Work out the finished part from the listing and answer in its coordinate system (mm). Give positions to 0.01 mm unless a question says otherwise; leave off trailing zeros. Loops run counter-clockwise (first coordinate to the right, second up) from the corner with the lowest first, then second, coordinate; pieces in that order, holes last. Notation, with made-up numbers: M -17,1 L -2,1 A14 ccw -2,18 Z; hole C 80,-15.75 d2. An arc over 180 degrees is marked long. Answer as a JSON object with one key per item and string values. Group by question number.
Autodesk Inventor part; units mm, degrees
ref_plane "YZ Plane" through (0, 0, 0) normal (1, 0, 0) x (0, 1, 0)
ref_plane "XZ Plane" through (0, 0, 0) normal (0, 1, 0) x (-1, 0, 0)
ref_plane "XY Plane" through (0, 0, 0) normal (0, 0, 1) x (1, 0, 0)
sketch "Sketch1" plane through (0, 0, 0) normal (0, 1, 0) x (-1, 0, 0)
  line L0 (-50, 50) -> (50, 50)
  line L1 (50, 50) -> (50, -50)
  line L2 (50, -50) -> (-50, -50)
  line L3 (-50, -50) -> (-50, 50)
  line L4 (-50, 50) -> (50, -50) construction
  line L5 (50, 50) -> (-50, -50) construction
  point P0 (0, 0)
  dimension "d0" = 100
  dimension "d1" = 100
extrude "Extrusion1" add sketch "Sketch1" along normal blind 3
sketch "Sketch2" plane through (0, 3, 0) normal (0, 1, 0) x (1, 0, 0)
  point P0 (0, 0)
  point P1 (0, 0)
hole "Hole1" at (0, 3, 0) direction (0, -1, 0) diameter 76.3 end through all
sketch "Sketch3" plane through (0, 3, 0) normal (0, 1, 0) x (1, 0, 0)
  line L0 (-50, -50) -> (50, -50)
  line L1 (-50, 50) -> (-50, -50)
  point P0 (0, 0)
  point P1 (-37.5, -37.5)
  point P2 (37.5, -37.5)
  point P3 (0, 0)
  point P4 (37.5, 37.5)
  point P5 (0, 0)
  point P6 (-37.5, 37.5)
  point P7 (0, 0)
  dimension "d18" = 12.5
  dimension "d19" = 12.5
  dimension "d22" = 360
hole "Hole2" at (-37.5, 3, 37.5) at (-37.5, 3, -37.5) at (37.5, 3, -37.5) at (37.5, 3, 37.5) direction (0, -1, 0) diameter 5 end through all
properties part number "Plant Panel" material "Aluminum 6061"
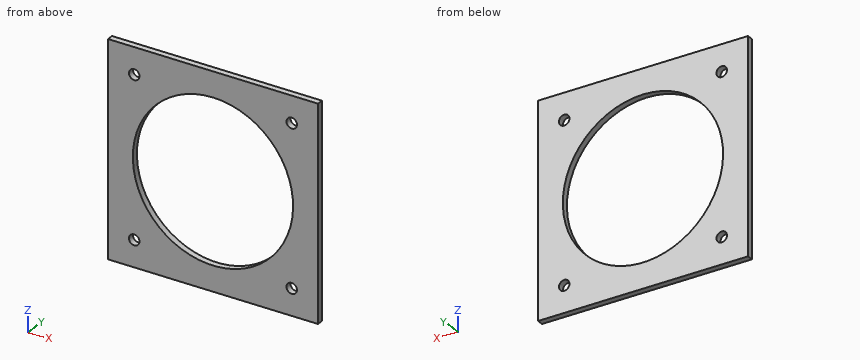
Item 1: A cutting plane is placed at B-B (x = 0). Determine the outline of the cut face in (y, z).
Item 2: A cutting plane is placed at A-A (z = 32.5). Determine the outline of the cut face in (x, y).
Item 3: Find the intervals of material crossed by probe 1 along X at (y, z) = (0.8, 39.5); probe 2 along X at (y, z) = (2.6, 0); probe 3 along X at (y, z) = (2, 13.5), in increasing order. Write a range as [from, to].
Item 4: A cutting plane is placed at C-C (y = 0.75). Determine the outline of the cut face in (x, z).
The answers:
{
 "1": {"outline": "M 0,-50 L 3,-50 L 3,-38.15 L 0,-38.15 Z; M 0,38.15 L 3,38.15 L 3,50 L 0,50 Z"},
 "2": {"outline": "M -50,0 L -19.98,0 L -19.98,3 L -50,3 Z; M 19.98,0 L 50,0 L 50,3 L 19.98,3 Z"},
 "3": {"probe 1": "x = [-50, -39], [-36, 36], [39, 50]", "probe 2": "x = [-50, -38.15], [38.15, 50]", "probe 3": "x = [-50, -35.68], [35.68, 50]"},
 "4": {"outline": "M -50,-50 L 50,-50 L 50,50 L -50,50 Z; hole C -37.5,-37.5 d5; hole C -37.5,37.5 d5; hole C 0,0 d76.3; hole C 37.5,-37.5 d5; hole C 37.5,37.5 d5"}
}
